from build123d import *

# Parameters (mm, degrees)
SKETCH2_R           = 5
SKETCH2_R_2         = 1.6
BOSS_EXTRUDE1_DEPTH = 5
BOSS_EXTRUDE2_DEPTH = 1.45


with BuildPart() as part:
    # Sketch2 → Boss-Extrude1 (new body)
    with BuildSketch(Plane.XY):
        Circle(SKETCH2_R)
        Circle(SKETCH2_R_2, mode=Mode.SUBTRACT)
    extrude(amount=BOSS_EXTRUDE1_DEPTH)

    # Sketch3 → Boss-Extrude2 (add)
    with BuildSketch(Plane.XY.offset(5)):
        with BuildLine():
            Line((0, 1.576678565), (0, 5))
            ThreePointArc((0, 5), (-5, 0), (0, -5))
            Line((0, -5), (0, -1.576678565))
            ThreePointArc((0, -1.576678565), (-1.576678565, 0), (0, 1.576678565))
        make_face()
    extrude(amount=BOSS_EXTRUDE2_DEPTH)


solid = part.part
Could you check a few things on this model? Use its own coordinates, in mm. A direction names the side the tool comes from. Give positions to 0.01 mm unless a question says otherwise; leave off trailing zeros. Loops run counter-clockwise (first coordinate to the right, second up) from the corner with the lowest first, then second, coordinate; pieces in that order, holes last. Notation, with made-up numbers: (46, -23.75) -> (105, -23.75) arc R10 ccw to (105, -17.75) -> close; hole circle Ø8 at (-33, 14.25). An arc over 180 degrees is marked (long way). Return JSON: item names as keys, results as strings.
Item 1: We'd pull the mould along Y, two halves only. Please class faces 1 (the flat face through (-3, 0, 6.45)), 2 (the cylindrical face through (-1.576, -0.035, 5.715)), 3 (the cylindrical face through (-5, 0, 3)): +Y half, -Y half, draft (parallel to the pull), parting line (faces both ways), or undercut.
Geometry results:
{"face 1": "draft", "face 2": "undercut", "face 3": "parting line"}
Item 2: I'm going to push flat-ended pins straight in: pin 1 (5.5 mm diameter, centred on x = 3.5, y = -0.5, fed in from +Z); pin 2 (3 mm diameter, centred on x = 1, z = 2, fed in from -Y); pin 3 (1.9 mm diameter, centred on x = 0, y = 0, fed in from +Z); pin 4 (0.7 mm diameter, centred on y = 3.5, z = 5.5, fed in from +X). Where does each tip first touch, or does it pass through?
Geometry results:
{"pin 1": "stops at z = 5", "pin 2": "stops at y = -5", "pin 3": "passes through", "pin 4": "stops at x = 0"}
Item 3: Which directions (+Z, -Z, +X, -X, +Y, -Y) give clear straight access to the entire face, cutting with the end or side of a thin tool? Please do faces 4 (the flat face through (2, 0, 5)), 5 (the cylindrical face through (-1.27, -0.97, 2.46)), 6 (the flat face through (2, 0, 0)).
Geometry results:
{"face 4": "+Z, +X, +Y, -Y", "face 5": "-Z", "face 6": "-Z, +X, -X, +Y, -Y"}
Item 4: If we section it at C-C on z = 3.25: List the corners of the cut face in (x, y) for me.
Geometry results:
{"outline": "circle Ø10 at (0, 0); hole circle Ø3.2 at (0, 0)"}
Item 5: If we section it at D-D on y = 4.5: List the corners of the cut face in (x, z) for me.
Geometry results:
{"outline": "(-2.18, 0) -> (2.18, 0) -> (2.18, 5) -> (0, 5) -> (0, 6.45) -> (-2.18, 6.45) -> close"}
Item 6: I need wall thicknesses on L1, parallel to Y at x = 0, z = 2; L2, parallel to Z at x = 2.5, y = 1. Which ranges of each line are inside material? Lowest first, please. Write a range as from..to.
Geometry results:
{"L1": "y = -5..-1.6, 1.6..5", "L2": "z = 0..5"}
Item 7: If we section it at B-B on x = 0.5: List the corners of the cut face in (y, z) for me, plus the area to 3 significant figures.
Geometry results:
{"outline": "(-4.97, 0) -> (-1.52, 0) -> (-1.52, 5) -> (-4.97, 5) -> close; (1.52, 0) -> (4.97, 0) -> (4.97, 5) -> (1.52, 5) -> close", "area": "34.6 mm²"}
